Input: part model. Units: mm. Frame: model coordinates. Face numbers are marked on the shaded views. A direction names the side the tool comes from. Coordinates: 2 decimals unless noted, no trailing zeros. Loops run counter-clockwise (first coordinate to the right, second up) from the corner with the lowest first, then second, coordinate; pieces in that order, holes last. Notation, with made-up numbers: (-25, -25) -> (14, -25) arc R11 ccw to (14, -18) -> close; hole circle Ø8 at (9, -16). An arc over 180 degrees is marked (long way). Put each result on its own line as item: value. Start each with the question number.
1) Pull-direction query (Y, two-part tool) for the marked faces 5, 6 and 7; classes: pulls with the +Y half, pulls with the -Y half, needs draft (parallel to the pull), parting line crosses it, or undercut.
2) Set-up query: the marked faces 1, 2, 3 and 4. Return all of +Z, -Z, +X, -X, +Y, -Y with unobstructed straight access to the full face (end or side cutting, diameter ignored); none if empty.
3) Contact query for flat-ended pins moving along their axis: P1, Ø4.5, axis at x = -3.5, z = 1.5, coming from the -Y side; P2, Ø3.5, axis at x = 31.9, y = -18.42, coming from the -Z side; P3, Ø4, axis at y = 17, z = 30.5, coming from the +X side; P4, Ø3, axis at y = 9, z = 3, coming from the +X side. Output: stop coordinate, or through.
4) Cut plane A-A (y = 0). Return the cut outline in (x, z), plus the area to 3 significant figures.
5) Material intervals for L1, parallel to X at y = 10.5, z = 6; L2, parallel to Z at x = -20, y = -8; L3, parallel to Y at x = 21, z = 23.5, sorted ascending.
from build123d import *

# Parameters (mm, degrees)
SKETCH1_R                 = 30.95625
BOSS_EXTRUDE1_DEPTH       = 50.8
CUT_EXTRUDE1_DEPTH        = 3.9624
CUT_EXTRUDE2_DEPTH        = 86.860858779
CUT_EXTRUDE2_DEPTH_BACK   = 86.860858779
SKETCH4_R                 = 19.05
CUT_EXTRUDE3_DEPTH        = 62.40755008
SKETCH6_R                 = 23.8125
CUT_EXTRUDE4_DEPTH        = 44.45
F_4_40_TAPPED_HOLE1_D     = 2.2606
F_4_40_TAPPED_HOLE1_DEPTH = 7.62
F_4_40_TAPPED_HOLE1_TIP   = 0.679152758
SKETCH10_R                = 40.48125
BOSS_EXTRUDE3_DEPTH       = 4.7625
FILLET1_R                 = 5.08
CIRPATTERN1_COUNT         = 2
CIRPATTERN1_ANGLE         = 120
SKETCH15_R                = 3.9624
CUT_EXTRUDE5_DEPTH        = 5.08


with BuildPart() as part:
    # Sketch1 → Boss-Extrude1 (new body)
    with BuildSketch(Plane.XY):
        Circle(SKETCH1_R)
    extrude(amount=BOSS_EXTRUDE1_DEPTH)

    # Sketch2 → Cut-Extrude1 (cut)
    with BuildSketch(Plane(origin=(0, 0, 0), x_dir=(-1, 0, 0), z_dir=(0, 0, -1))):
        with BuildLine():
            Line((-18.3261, -22.2885), (18.3261, -22.2885))
            ThreePointArc((18.3261, -22.2885), (21.12793991, -21.12793991), (22.2885, -18.3261))
            Line((22.2885, -18.3261), (22.2885, 18.3261))
            ThreePointArc((22.2885, 18.3261), (21.12793991, 21.12793991), (18.3261, 22.2885))
            Line((18.3261, 22.2885), (-18.3261, 22.2885))
            ThreePointArc((-18.3261, 22.2885), (-21.12793991, 21.12793991), (-22.2885, 18.3261))
            Line((-22.2885, 18.3261), (-22.2885, -18.3261))
            ThreePointArc((-22.2885, -18.3261), (-21.12793991, -21.12793991), (-18.3261, -22.2885))
        make_face()
    extrude(amount=-CUT_EXTRUDE1_DEPTH, mode=Mode.SUBTRACT)

    # Sketch3 → Cut-Extrude2 (cut, two sides: drawn at the far end of the back side and taken through both)
    with BuildSketch(Plane(origin=(30.95625, 0, 0), x_dir=(0.14780941112961093, 0, -0.9890158633619168), z_dir=(0.9890158633619168, 0, 0.14780941112961093)).offset(-CUT_EXTRUDE2_DEPTH_BACK)):
        with BuildLine():
            Line((-48.467631025, 25.4), (-4.575625083, 30.95625))
            Line((-4.575625083, 30.95625), (-67.517631025, 30.95625))
            Line((-67.517631025, 30.95625), (-67.517631025, -30.95625))
            Line((-67.517631025, -30.95625), (-4.575625083, -30.95625))
            Line((-4.575625083, -30.95625), (-48.467631025, -25.4))
            ThreePointArc((-48.467631025, -25.4), (-23.067631025, 0), (-48.467631025, 25.4))
        make_face()
    extrude(amount=CUT_EXTRUDE2_DEPTH + CUT_EXTRUDE2_DEPTH_BACK, mode=Mode.SUBTRACT)

    # Sketch4 → Cut-Extrude3 (cut, through all)
    with BuildSketch(Plane(origin=(0, 0, 3.9624), x_dir=(-1, 0, 0), z_dir=(0, 0, -1))):
        Circle(SKETCH4_R)
    extrude(amount=-CUT_EXTRUDE3_DEPTH, mode=Mode.SUBTRACT)

    # Sketch6 → Cut-Extrude4 (cut)
    with BuildSketch(Plane.XY.offset(50.8)):
        Circle(SKETCH6_R)
    extrude(amount=-CUT_EXTRUDE4_DEPTH, mode=Mode.SUBTRACT)

    # #4-40 Tapped Hole1
    with Locations(Plane(origin=(0, 0, 3.9624), x_dir=(-1, 0, 0), z_dir=(0, 0, -1))):
        with Locations((-18.2626, 18.2626), (18.2626, 18.2626), (18.2626, -18.2626), (-18.2626, -18.2626)):
            Hole(F_4_40_TAPPED_HOLE1_D / 2, depth=F_4_40_TAPPED_HOLE1_DEPTH)
            with Locations((0, 0, -(F_4_40_TAPPED_HOLE1_DEPTH + F_4_40_TAPPED_HOLE1_TIP / 2))):  # 118° drill point
                Cone(0, F_4_40_TAPPED_HOLE1_D / 2, F_4_40_TAPPED_HOLE1_TIP, mode=Mode.SUBTRACT)

    # Sketch10 → Boss-Extrude3 (add)
    with BuildSketch(Plane(origin=(0, 0, 0), x_dir=(-1, 0, 0), z_dir=(0, 0, -1))):
        Circle(SKETCH10_R)
        with BuildLine():
            Line((-17.695463093, 25.4), (17.695463093, 25.4))
            ThreePointArc((17.695463093, 25.4), (30.95625, 0), (17.695463093, -25.4))
            Line((17.695463093, -25.4), (-17.695463093, -25.4))
            ThreePointArc((-17.695463093, -25.4), (-30.95625, 0), (-17.695463093, 25.4))
        make_face(mode=Mode.SUBTRACT)
    extrude(amount=-BOSS_EXTRUDE3_DEPTH)

    # Fillet1
    fillet1_edges = [part.edges().sort_by_distance(p)[0] for p in [
        (30.95625, 0, 4.7625),
        (-30.95625, 0, 4.7625),
        (-0.567868867, -30.349366054, 4.7625),
        (-0.567868867, 30.349366054, 4.7625),
    ]]
    fillet(fillet1_edges, radius=FILLET1_R)

    # Sketch13 → #8 Clearance Hole1 (revolve, cut)
    with BuildSketch(Plane(origin=(-31.895715621, 18.415, 4.7625), x_dir=(0, -1, 0), z_dir=(1, 0, 0))):
        Polygon((0, 0), (0, 26.750674586), (2.2479, 25.4), (2.2479, 0), align=None)
    f_8_clearance_hole1 = revolve(axis=Axis((-31.895715621, 18.415, 11.1125), (0, 0, -1)), mode=Mode.SUBTRACT)

    # CirPattern1: #8 Clearance Hole1 ×2 about axis
    cirpattern1_axis = Axis((0, 0, 4.7625), (0, 0, -1))
    for i in range(1, CIRPATTERN1_COUNT):
        add(f_8_clearance_hole1.rotate(cirpattern1_axis, i * CIRPATTERN1_ANGLE / (CIRPATTERN1_COUNT - 1)), mode=Mode.SUBTRACT)

    # Mirror1: #8 Clearance Hole1 across plane
    add(f_8_clearance_hole1.mirror(Plane.ZX), mode=Mode.SUBTRACT)

    # Mirror1 copy 1 sketch → Mirror1 copy 1 (revolve, cut)
    with BuildSketch(Plane(origin=(31.895715621, -18.415, 4.7625), x_dir=(-0.866025403784436, -0.5000000000000044, 0), z_dir=(-0.5000000000000044, 0.866025403784436, 0))):
        Polygon((0, 0), (0, -26.750674586), (2.2479, -25.4), (2.2479, 0), align=None)
    revolve(axis=Axis((31.895715621, -18.415, 11.1125), (0, 0, 1)), mode=Mode.SUBTRACT)

    # Sketch15 → Cut-Extrude5 (cut)
    with BuildSketch(Plane.XY.offset(9.8425)):
        with Locations((-31.895715621, 18.415)):
            Circle(SKETCH15_R)
        with Locations((31.895715621, 18.415)):
            Circle(SKETCH15_R)
        with Locations((31.895715621, -18.415)):
            Circle(SKETCH15_R)
        with Locations((-31.895715621, -18.415)):
            Circle(SKETCH15_R)
    extrude(amount=-CUT_EXTRUDE5_DEPTH, mode=Mode.SUBTRACT)


solid = part.part
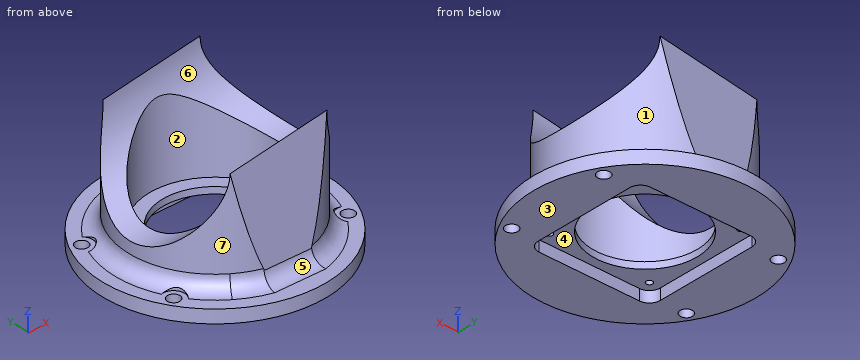
Results found:
1. face 5: pulls with the -Y half
1. face 6: undercut
1. face 7: parting line crosses it
2. face 1: +Z, +X
2. face 2: +Z
2. face 3: -Z, +X, -X, +Y, -Y
2. face 4: -Z
3. P1: stops at y = -40.46
3. P2: passes through
3. P3: stops at x = 26.31
3. P4: stops at x = 39.78
4. outline: (-40.48, 0) -> (-22.29, 0) -> (-22.29, 3.96) -> (-19.05, 3.96) -> (-19.05, 6.35) -> (-23.81, 6.35) -> (-23.81, 15.14) -> (-30.96, 14.07) -> (-30.96, 9.84) arc R5.08 cw to (-36.04, 4.76) -> (-40.48, 4.76) -> close; (19.05, 3.96) -> (22.29, 3.96) -> (22.29, 0) -> (40.48, 0) -> (40.48, 4.76) -> (36.04, 4.76) arc R5.08 cw to (30.96, 9.84) -> (30.96, 23.32) -> (23.81, 22.26) -> (23.81, 6.35) -> (19.05, 6.35) -> close
4. area: 404 mm2
5. L1: x = -30.98 to -15.9, 15.9 to 30.98
5. L2: z = 3.96 to 6.35
5. L3: y = -22.74 to -11.23, 11.23 to 22.74
